```python
from build123d import *

# Parameters (mm, degrees)
F0_W     = 82.0386651903
F0_H     = 68.6869425699
F1_DEPTH = 10.16
F3_D     = 5.08
F3_DEPTH = 12.7
F3_TIP   = 1.5261859723


with BuildPart() as f1:
    # F0 (on Front) → F1 (new body)
    with BuildSketch(Plane.XZ):
        with Locations((-19.4462044165, 23.5556685366)):
            Rectangle(F0_W, F0_H)
    extrude(amount=F1_DEPTH)

    # F3
    with Locations(Plane(origin=(0, 0, -10.7878027484), x_dir=(1, 0, 0), z_dir=(0, 0, -1))):
        with Locations((-17.4416806549, 5.4131019861)):
            Hole(F3_D / 2, depth=F3_DEPTH)
            with Locations((0, 0, -(F3_DEPTH + F3_TIP / 2))):  # 118° drill point
                Cone(0, F3_D / 2, F3_TIP, mode=Mode.SUBTRACT)


solid = f1.part
```
Here's how the part is built. I have some questions about the finished solid (model axes, mm). A direction names the side the tool comes from. Give positions to 0.01 mm unless a question says otherwise; leave off trailing zeros. Loops run counter-clockwise (first coordinate to the right, second up) from the corner with the lowest first, then second, coordinate; pieces in that order, holes last. Notation, with made-up numbers: (20, 51.5) -> (62, 51.5) arc R22 ccw to (62, 83.5) -> close; hole circle Ø7 at (56, 21.25). An arc over 180 degrees is marked (long way). Use one line per item in the form item = value. Start each with the question number.
1) Imagine slicing it at A-A (z = -3). Please give me the cut outline in (x, y), then the cut area to 3 significant figures.
2) Please list where this line runs through material, in increasing order: line 1 along Z through (x, y) = (-18.5, -6).
3) Which directions (+Z, -Z, +X, -X, +Y, -Y) give clear straight access to the entire face, cutting with the end or side of a thin tool? Please do faces 1 (the face through (-19.79, -4.44, -4.35)), 2 (the face through (-60.466, -5, 23)).
4) Thinking about a two-plate mould opening in X: for faces 3 (the face through (-17.767, -5.711, 3.173)), 4 (the face through (21.573, -5, 23)), 5 (the face through (-20, 0, 24)), which applies, +X half, -X half, draft (parallel to the pull), parting line (faces both ways), or undercut?
Check values:
q1.outline = (-60.47, -10.16) -> (21.57, -10.16) -> (21.57, 0) -> (-60.47, 0) -> close; hole circle Ø5.08 at (-17.44, -5.41)
q1.area = 813 mm^2
q2.line_1 = 2.71 to 57.9
q3.face_1 = -Z
q3.face_2 = +Z, -Z, -X, +Y, -Y
q4.face_3 = undercut
q4.face_4 = +X half
q4.face_5 = draft
